```python
from build123d import *

# Parameters (mm, degrees)
SKETCH2_R           = 2.5
BOSS_EXTRUDE1_DEPTH = 5
BOSS_EXTRUDE2_START = -10
SKETCH3_R           = 2.5
SKETCH3_R_2         = 0.5
BOSS_EXTRUDE2_DEPTH = 10
SKETCH4_R           = 2.5
SKETCH4_R_2         = 0.5
BOSS_EXTRUDE3_DEPTH = 8
SKETCH5_R           = 2.5
BOSS_EXTRUDE4_DEPTH = 5


with BuildPart() as part:
    # Sketch2 → Boss-Extrude1 (new body)
    with BuildSketch(Plane.XY):
        with BuildLine():
            Line((-24, 4), (0, 4))
            ThreePointArc((0, 4), (2.294305745, 3.276608177), (3.758770483, 1.368080573))
            Line((3.758770483, 1.368080573), (6.323921558, -5.679614083))
            ThreePointArc((6.323921558, -5.679614083), (5.517602021, -9.746404239), (1.539439822, -10.913948195))
            Line((1.539439822, -10.913948195), (-25.025711253, -3.866253539))
            ThreePointArc((-25.025711253, -3.866253539), (-27.966422453, 0.51719718), (-24, 4))
        make_face()
        with Locations((-24, 0)):
            Circle(SKETCH2_R, mode=Mode.SUBTRACT)
        Circle(SKETCH2_R, mode=Mode.SUBTRACT)
        with Locations((2.565151075, -7.047694656)):
            Circle(SKETCH2_R, mode=Mode.SUBTRACT)
    extrude(amount=BOSS_EXTRUDE1_DEPTH)

    # Sketch3 → Boss-Extrude2 (add)
    with BuildSketch(Plane.XY.offset(5).offset(BOSS_EXTRUDE2_START)):
        Circle(SKETCH3_R)
        Circle(SKETCH3_R_2, mode=Mode.SUBTRACT)
    extrude(amount=BOSS_EXTRUDE2_DEPTH)

    # Sketch4 → Boss-Extrude3 (add)
    with BuildSketch(Plane(origin=(0, 0, 0), x_dir=(-1, 0, 0), z_dir=(0, 0, -1))):
        with Locations((-2.565151075, -7.047694656)):
            Circle(SKETCH4_R)
        with Locations((-2.565151075, -7.047694656)):
            Circle(SKETCH4_R_2, mode=Mode.SUBTRACT)
    extrude(amount=-BOSS_EXTRUDE3_DEPTH)

    # Sketch5 → Boss-Extrude4 (add)
    with BuildSketch(Plane(origin=(0, 0, 0), x_dir=(-1, 0, 0), z_dir=(0, 0, -1))):
        with Locations((24, 0)):
            Circle(SKETCH5_R)
    extrude(amount=-BOSS_EXTRUDE4_DEPTH)


solid = part.part
```
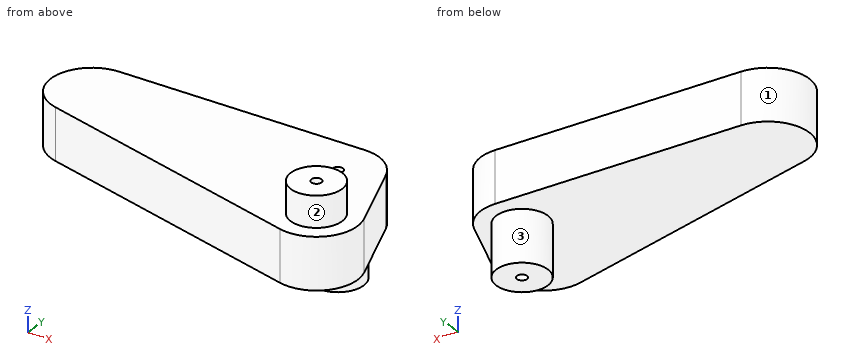
Build history of the part. All positions in model axes, mm. Face numbers are marked on the shaded views. A direction names the side the tool comes from. Give positions to 0.01 mm unless a question says otherwise; leave off trailing zeros. Order: outer loops, then holes, each group sorted by start corner. A loop starts at its lowest first (then second) coordinate and runs counter-clockwise, first axis right, second up. Notation, with made-up numbers: M -7.75,34 L 26.25,34 A15 ccw 26.25,56 Z; hole C 50.25,47.5 d9. An arc over 180 degrees is marked long. Write item = value, one per line. Start each with the question number.
(1) Pin check, flat tips, straight feed: pin 1 Ø5 at (x, y) = (-10.5, 0) entering from +Z; pin 2 Ø1 at (y, z) = (-1.5, -3) entering from -X; pin 3 Ø1.5 at (y, z) = (-6, 4) entering from +X. Stop position of each tip, or through.
(2) Slice it at B-B on z = 1.5. Write the cut outline in (x, y), plus the area to 3 significant figures.
(3) Probe L1, parallel to Y at x = 0, z = -0.25; L2, parallel to Z at x = -6.5, y = 0; L3, parallel to Z at x = -1.5, y = 0.5. List the from-to ranges inside material, lowest first. Write a range as [from, to].
(4) Slice it at C-C on x = -22.5. Write the cut outline in (y, z).
(5) Which spindle directions (+Z, -Z, +X, -X, +Y, -Y) get a long thin tool onto all of the face, cutting with end or side? Do the marked faces 1, 2 and 3. Say none if no direction does.
(6) Slice it at D-D on y = 1.75. Write the cut outline in (x, z).
(7) Slice it at A-A on y = 0. Write the cut outline in (x, z), plus the area to 3 significant figures.
Responses:
q1.pin_1 = 5
q1.pin_2 = -2.29
q1.pin_3 = 6.55
q2.outline = M -25.03,-3.87 L 1.54,-10.91 A4 ccw 6.32,-5.68 L 3.76,1.37 A4 ccw 0,4 L -24,4 A4 ccw Z; hole C 0,0 d1; hole C 2.57,-7.05 d1
q2.area = 369 mm2
q3.L1 = [-2.5, -0.5], [0.5, 2.5]
q3.L2 = [0, 5]
q3.L3 = [-5, 5]
q4.outline = M -4.54,0 L 4,0 L 4,5 L -4.54,5 Z
q5.face_1 = +Z, -Z, -X
q5.face_2 = +Z
q5.face_3 = -Z
q6.outline = M -27.6,0 L -1.79,0 L -1.79,-5 L 1.79,-5 L 1.79,0 L 3.6,0 L 3.6,5 L -27.6,5 Z
q7.outline = M -28,0 L -2.5,0 L -2.5,-5 L -0.5,-5 L -0.5,5 L -28,5 Z; M 0.5,-5 L 2.5,-5 L 2.5,0 L 4.26,0 L 4.26,5 L 0.5,5 Z
q7.area = 176 mm2
